Autodesk Inventor part; units mm, degrees
ref_plane "YZ Plane" through (0, 0, 0) normal (1, 0, 0) x (0, 1, 0)
ref_plane "XZ Plane" through (0, 0, 0) normal (0, 1, 0) x (-1, 0, 0)
ref_plane "XY Plane" through (0, 0, 0) normal (0, 0, 1) x (1, 0, 0)
sketch "Sketch2" plane through (0, 0, 0) normal (0, 1, 0) x (-1, 0, 0)
  line L0 (2.8786, -13.004) -> (2.8786, -16.004)
  line L1 (-3.1214, -13.004) -> (-3.1214, -16.004)
  line L2 (10.3786, -16.004) -> (10.3786, -13.004) construction
  line L3 (7.3786, -13.004) -> (7.3786, -16.004)
  line L4 (-7.6214, -16.004) -> (-7.6214, -13.004)
  line L5 (-10.6214, -13.004) -> (-10.6214, -16.004)
  line L6 (15.3786, -13.004) -> (15.3786, 12.596)
  line L7 (10.3786, 15.596) -> (10.3786, 12.5963)
  line L8 (7.3786, 12.596) -> (7.3786, 15.596)
  line L9 (2.8786, 15.7558) -> (2.8786, 12.596)
  line L10 (-3.1214, 12.7558) -> (-3.1214, 15.7558)
  line L11 (-7.6214, 15.7558) -> (-7.6214, 12.7558)
  line L12 (-10.6214, 12.596) -> (-10.6214, 15.7558)
  line L13 (10.3786, -16.004) -> (10.3786, -13.004)
  line L14 (15.3786, -13.004) -> (10.3786, -13.004)
  line L15 (10.3786, -16.004) -> (7.3786, -16.004)
  line L16 (7.3786, -13.004) -> (2.8786, -13.004)
  line L17 (2.8786, -16.004) -> (-3.1214, -16.004)
  line L18 (-3.1214, -13.004) -> (-7.6214, -13.004)
  line L19 (-7.6214, -16.004) -> (-10.6214, -16.004)
  line L20 (-10.6214, -13.004) -> (-15.6214, -13.004)
  line L21 (-15.6214, 12.596) -> (-10.6214, 12.596)
  line L22 (-10.6214, 15.7558) -> (-7.6214, 15.7558)
  line L23 (-7.6214, 12.7558) -> (-3.1214, 12.7558)
  line L24 (-3.1214, 15.7558) -> (2.8786, 15.7558)
  line L25 (2.8786, 12.596) -> (7.3786, 12.596)
  line L26 (7.3786, 15.596) -> (10.3786, 15.596)
  line L27 (10.3786, 12.5963) -> (15.3786, 12.596)
  line L28 (-15.6214, 12.596) -> (-15.6214, -13.004)
  line L29 (15.3786, -0.204) -> (-15.6214, -0.204) construction
  line L30 (7.3786, -13.004) -> (7.3786, -0.204) construction
  line L31 (7.3786, -0.204) -> (7.3786, 12.596) construction
  line L32 (2.8786, -10.204) -> (-3.1214, -10.204)
  line L33 (-3.1214, -10.204) -> (-3.1214, -7.204)
  line L34 (-3.1214, -7.204) -> (2.8786, -7.204)
  line L35 (2.8786, -7.204) -> (2.8786, -10.204)
  line L36 (2.8786, 6.796) -> (-3.1214, 6.796)
  line L37 (-3.1214, 6.796) -> (-3.1214, 9.796)
  line L38 (-3.1214, 9.796) -> (2.8786, 9.796)
  line L39 (2.8786, 9.796) -> (2.8786, 6.796)
  dimension "d14" = 3
  dimension "d15" = 3
  dimension "d16" = 6
  dimension "d17" = 31
  dimension "d18" = 4.5
  dimension "d19" = 25.6
  dimension "d39" = 6
  dimension "d40" = 3
  dimension "d41" = 7
  dimension "d42" = 6
  dimension "d43" = 3
  dimension "d44" = 7
extrude "Extrusion1" add sketch "Sketch2" along normal blind 3 contours L0 L17 L1 L18 L4 L19 L5 L20 L28 L21 L12 L22 L11 L23 L10 L24 L9 L25 L8 L26 L7 L27 L6 L14 L13 L15 L3 L16 | L32 L33 L34 L35 | L36 L37 L38 L39
extrude "Extrusion2" cut sketch "Sketch2" along normal up to next contours L36 L37 L38 L39
extrude "Extrusion3" cut sketch "Sketch2" along normal up to next contours L32 L33 L34 L35
properties part number "part_plunger_handle_side2"
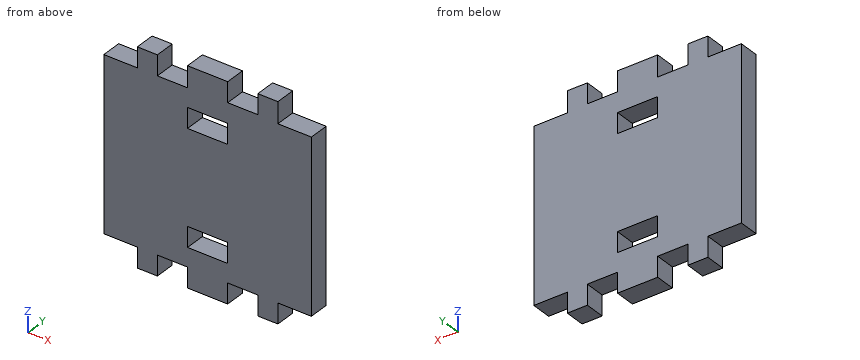
Here's how the part is built. I have some questions about the finished solid (model axes, mm). Round coordinates to 2 decimals unless told otherwise and drop trailing zeros. Write each loop counter-clockwise with the first axis right and the second up, starting at its lowest first coordinate (ties: lowest second). Pieces come first, ordered by that corner, then holes. Notation, with made-up numbers: (55, 18.5) -> (102, 18.5) arc R14 ccw to (102, 33.5) -> close; hole circle Ø2 at (87.5, -39). An arc over 180 degrees is marked (long way). One line per item, written item: value.
1) Suppose I cut it at B-B on z = 8.5. List the corners of the cut face in (x, y) for me.
Filled sheet:
outline: (-15.38, 0) -> (-2.88, 0) -> (-2.88, 3) -> (-15.38, 3) -> close; (3.12, 0) -> (15.62, 0) -> (15.62, 3) -> (3.12, 3) -> close
2) I'm going to push flat-ended pins straight in: pin 1 Ø0.9 at (y, z) = (1.5, 13.5) entering from +X; pin 2 Ø0.9 at (y, z) = (1.5, -15) entering from -X. Where does each tip first touch, or does it pass through?
Filled sheet:
pin 1: stops at x = 10.62
pin 2: stops at x = -10.38
3) Suppose I cut it at D-D on x = 4. List the corners of the cut face in (y, z) for me.
Filled sheet:
outline: (0, -13) -> (3, -13) -> (3, 12.76) -> (0, 12.76) -> close
4) Suppose I cut it at C-C on y = 0.55. Give the number of separate pieces and of enclosed holes in the cut face, plus the area to 3 significant figures.
Filled sheet:
separate pieces: 1
enclosed holes: 2
area: 832 mm2
5) Suppose I cut it at A-A on x = 0. List the corners of the cut face in (y, z) for me, plus the area to 3 significant figures.
Filled sheet:
outline: (0, -16) -> (3, -16) -> (3, -10.2) -> (0, -10.2) -> close; (0, -7.2) -> (3, -7.2) -> (3, 6.8) -> (0, 6.8) -> close; (0, 9.8) -> (3, 9.8) -> (3, 15.76) -> (0, 15.76) -> close
area: 77.3 mm2
6) If I drill on line 1 (Z direction, x = 0.5, y = 0.25); line 2 (X direction, y = 1.6, z = -14); line 3 (X direction, y = 1.3, z = 9.5), over which ranges is the centre line in solid material (lowest first)? Write a range as [from, to].
Filled sheet:
line 1: z = [-16, -10.2], [-7.2, 6.8], [9.8, 15.76]
line 2: x = [-10.38, -7.38], [-2.88, 3.12], [7.62, 10.62]
line 3: x = [-15.38, -2.88], [3.12, 15.62]
